Autodesk Inventor part; units mm, degrees
ref_plane "YZ Plane" through (0, 0, 0) normal (1, 0, 0) x (0, 1, 0)
ref_plane "XZ Plane" through (0, 0, 0) normal (0, 1, 0) x (-1, 0, 0)
ref_plane "XY Plane" through (0, 0, 0) normal (0, 0, 1) x (1, 0, 0)
sketch "Sketch1" plane through (0, 0, 0) normal (0, 0, 1) x (1, 0, 0)
  circle A0 centre (0, 0) radius 100
  line L0 (0, 100) -> (86.6025, 50)
  line L1 (86.6025, 50) -> (86.6025, -50)
  line L2 (86.6025, -50) -> (0, -100)
  line L3 (0, -100) -> (-86.6025, -50)
  line L4 (-86.6025, -50) -> (-86.6025, 50)
  line L5 (-86.6025, 50) -> (0, 100)
  circle A1 centre (0, 0) radius 50
  circle A2 centre (0, 0) radius 15
  circle A3 centre (0, 0) radius 6.35
  circle A4 centre (32.256, 0) radius 4
  circle A5 centre (-16.128, 27.9345) radius 4
  circle A6 centre (-16.128, -27.9345) radius 4
  dimension "d0" = 200
  dimension "d1" = 100
  dimension "d2" = 30
  dimension "d3" = 12.7
  dimension "d4" = 8
  dimension "d7" = 360
extrude "Plate1" add sketch "Sketch1" against normal blind 5 contours A1 | A2 | A3
extrude "Extrusion1" add sketch "Sketch1" along normal blind 37 contours A2
thread "Thread1"
equation "\"d9\" = Thickness"
equation "\"BendRadius\" = Thickness"
equation "\"BendReliefWidth\" = Thickness"
equation "\"BendReliefDepth\" = 0.5 * Thickness"
equation "\"TransitionRadius\" = BendRadius"
equation "\"JacobiRadiusSize\" = BendRadius"
equation "\"GapSize\" = Thickness"
properties part number "Test flange" material "Aluminum 6061"
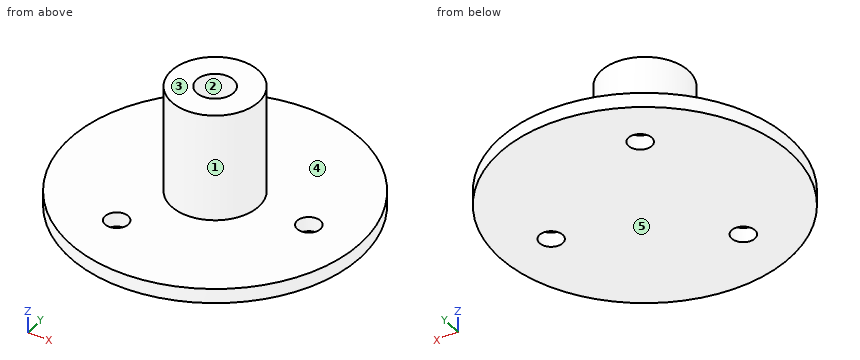
Can you work these out from the model? Positions are in its coordinate system, mm. Face numbers are marked on the shaded views. A direction names the side the tool comes from. Round coordinates to 2 decimals unless told otherwise and drop trailing zeros. Order: outer loops, then holes, each group sorted by start corner. A loop starts at its lowest first (then second) coordinate and runs counter-clockwise, first axis right, second up. Notation, with made-up numbers: (-30.75, 38.25) - (-11.75, 38.25) arc R28 ccw to (-11.75, 62.25) - close; hole circle Ø4 at (-4, 62). An arc over 180 degrees is marked (long way). Answer in a Markdown table with one row per item.
(1) Suppose I cut it at D-D, the plane x = -16.5. Please give me the cut outline in (y, z), plus the area to 3 significant figures.
From the geometry:
| item | result |
|---|---|
| outline | (-47.2, -5) - (-31.92, -5) - (-31.92, 0) - (-47.2, 0) - close; (-23.95, -5) - (23.95, -5) - (23.95, 0) - (-23.95, 0) - close; (31.92, -5) - (47.2, -5) - (47.2, 0) - (31.92, 0) - close |
| area | 392 mm2 |
(2) Suppose I cut it at A-A, the plane y = 0. Please give me the cut outline in (x, z), plus the area to 3 significant figures.
From the geometry:
| item | result |
|---|---|
| outline | (-50, -5) - (28.26, -5) - (28.26, 0) - (15, 0) - (15, 37) - (6.35, 37) - (6.35, 0) - (-6.35, 0) - (-6.35, 37) - (-15, 37) - (-15, 0) - (-50, 0) - close; (36.26, -5) - (50, -5) - (50, 0) - (36.26, 0) - close |
| area | 1,100 mm2 |
(3) Suppose I cut it at B-B, the plane x = 31. Please give me the cut outline in (y, z).
From the geometry:
| item | result |
|---|---|
| outline | (-39.23, -5) - (-3.8, -5) - (-3.8, 0) - (-39.23, 0) - close; (3.8, -5) - (39.23, -5) - (39.23, 0) - (3.8, 0) - close |
(4) Suppose I cut it at C-C, the plane z = 30. Please give me the cut outline in (x, y).
From the geometry:
| item | result |
|---|---|
| outline | circle Ø30 at (0, 0); hole circle Ø12.7 at (0, 0) |
(5) If we mould it in two halves opening along Y, with no side actions, what happens to the marked faces 1, 2 and 3? For each: released by +Y, released by -Y, zero draft, split by the parting line, or undercut.
From the geometry:
| item | result |
|---|---|
| face 1 | split by the parting line |
| face 2 | undercut |
| face 3 | zero draft |
(6) For P1, Ø1, axis at y = 5.5, z = 25, coming from the +X side; P2, Ø4, axis at x = -0.5, y = 1, coming from the +Z side; P3, Ø8, axis at x = 1.5, z = 20.5, coming from the +Y side; P4, Ø5, axis at x = 32.256, y = 0, coming from the -Z side, each with a flat end and sliding along its axis, tell me the tip position at first contact or that it passes through.
From the geometry:
| item | result |
|---|---|
| P1 | stops at x = 14.14 |
| P2 | stops at z = 0 |
| P3 | stops at y = 15 |
| P4 | passes through |
(7) Which directions (+Z, -Z, +X, -X, +Y, -Y) give clear straight access to the entire face, cutting with the end or side of a thin tool? Please do the marked faces 4 and 5.
From the geometry:
| item | result |
|---|---|
| face 4 | +Z |
| face 5 | -Z, +X, -X, +Y, -Y |
(8) Please list where these lines run through material, in increasing order: L1, parallel to Y at x = 0, z = 10; L2, parallel to Z at x = -6, y = 15.5; L3, parallel to X at y = -5, z = 9.5. Write a range as from..to.
From the geometry:
| item | result |
|---|---|
| L1 | y = -15..-6.35, 6.35..15 |
| L2 | z = -5..0 |
| L3 | x = -14.14..-3.91, 3.91..14.14 |
